from build123d import *

# Parameters (mm, degrees)
F1_DEPTH = 157.48
F2_R     = 25.233792
F3_DEPTH = 142.748
F5_DEPTH = 8.636
F6_R     = 1.660828
F7_DEPTH = 7.112


with BuildPart() as f1:
    # F0 (on Top) → F1 (new body)
    with BuildSketch(Plane.XY):
        Polygon((-8.753945, -81.124703), (74.44906, -33.394409), (54.765995, 60.485824), (-40.601814, 70.776703), (-79.859295, -16.743415), align=None)
    extrude(amount=F1_DEPTH)

    # F2 (on Top) → F3 (cut)
    with BuildSketch(Plane.XY):
        Circle(F2_R)
    extrude(amount=F3_DEPTH, mode=Mode.SUBTRACT)

    # F4 (on face) → F5 (join)
    with BuildSketch(Plane.XY.offset(157.48)):
        Polygon((2.463029, -4.001475), (4.696893, 0.132308), (2.233864, 4.133783), (-2.463029, 4.001475), (-4.696893, -0.132308), (-2.233864, -4.133783), align=None)
    extrude(amount=F5_DEPTH)

    # F6 (on face) → F7 (join)
    with BuildSketch(Plane.XY.offset(166.116)):
        Circle(F6_R)
    extrude(amount=F7_DEPTH)


solid = f1.part
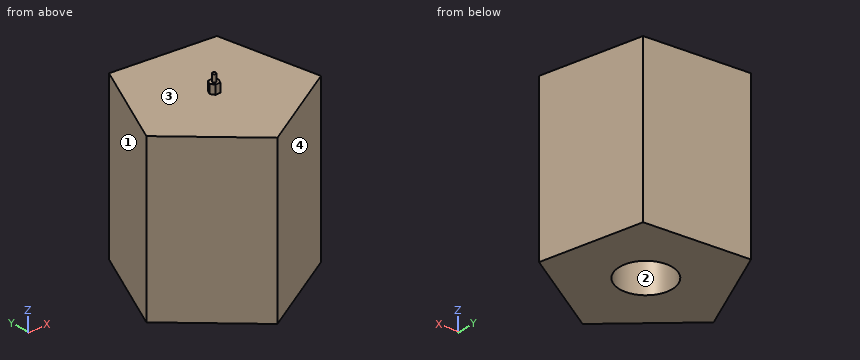
Build history of the part. All positions in model axes, mm. Face numbers are marked on the shaded views. Round coordinates to 2 decimals unless told otherwise and drop trailing zeros. Loops run counter-clockwise (first coordinate to the right, second up) from the corner with the lowest first, then second, coordinate; pieces in that order, holes last. Notation, with made-up numbers: (23, -29.75) -> (70, -29.75) arc R22 cw to (70, -12.75) -> close; hole circle Ø6 at (66, 27.25). An arc over 180 degrees is marked (long way). Answer in a Markdown table with one row per item.
Item 1: Pin check, flat tips, straight feed: pin 1 (5 mm diameter, centred on x = 15, z = 128, fed in from +Y); pin 2 (10 mm diameter, centred on x = -27.5, y = 8, fed in from +Z); pin 3 (8 mm diameter, centred on x = -54.5, z = 105.5, fed in from +Y). Stop position of each tip, or through.
Answers below:
| item | result |
|---|---|
| pin 1 | stops at y = 65.05 |
| pin 2 | stops at z = 157.48 |
| pin 3 | stops at y = 48.71 |
Item 2: Saw through at D-D (y = -47.5). Write the cut outline in (x, z).
Answers below:
| item | result |
|---|---|
| outline | (-45.89, 0) -> (49.86, 0) -> (49.86, 157.48) -> (-45.89, 157.48) -> close |
Item 3: Saw through at B-B (x = -23). Write the cut outline in (y, z), and give its area (3 significant figures).
Answers below:
| item | result |
|---|---|
| outline | (-68.23, 0) -> (-10.38, 0) -> (-10.38, 142.75) -> (10.38, 142.75) -> (10.38, 0) -> (68.88, 0) -> (68.88, 157.48) -> (-68.23, 157.48) -> close |
| area | 18,600 mm² |
Item 4: Mould opens along X. For the marked faces 1, 2, 3 and 4 say: +X half, -X half, draft (parallel to the pull), parting line (faces both ways), or undercut.
Answers below:
| item | result |
|---|---|
| face 1 | -X half |
| face 2 | undercut |
| face 3 | draft |
| face 4 | +X half |
Item 5: Drill centre lines: L1, parallel to Z at x = 34, y = -55.5; L2, parallel to X at y = -17, z = 106; L3, parallel to X at y = 23, z = 140. Where is each one in solid material? Low to high. Write a range as [from, to].
Answers below:
| item | result |
|---|---|
| L1 | z = [0, 157.48] |
| L2 | x = [-79.58, -18.65], [18.65, 71.01] |
| L3 | x = [-62.03, -10.38], [10.38, 62.63] |
Item 6: Saw through at A-A (z = 120). Write the cut outline in (x, y).
Answers below:
| item | result |
|---|---|
| outline | (-79.86, -16.74) -> (-8.75, -81.12) -> (74.45, -33.39) -> (54.77, 60.49) -> (-40.6, 70.78) -> close; hole circle Ø50.47 at (0, 0) |
Item 7: Saw through at C-C (z = 148). Write the cut outline in (x, y), and give its area (3 significant figures).
Answers below:
| item | result |
|---|---|
| outline | (-79.86, -16.74) -> (-8.75, -81.12) -> (74.45, -33.39) -> (54.77, 60.49) -> (-40.6, 70.78) -> close |
| area | 15,800 mm² |
